Autodesk Inventor part; units mm, degrees
ref_plane "Arbeitsebene1" through (1.75, 0, 2.75) normal (0, 0, 1) x (1, 0, 0)
ref_plane "YZ Plane" through (0, 0, 0) normal (1, 0, 0) x (0, 1, 0)
ref_plane "XZ Plane" through (0, 0, 0) normal (0, 1, 0) x (-1, 0, 0)
sketch "Skizze1" plane through (0, 0, 0) normal (0, 0, 1) x (1, 0, 0)
  line L0 (-3.4, 0) -> (20.4, 0)
  line L1 (0, -0.55) -> (0, 3.3)
  line L2 (0, 2.75) -> (3.5, 2.75)
  line L3 (3.5, 2.75) -> (3.5, 2.5)
  line L4 (3.5, 2.5) -> (17, 2.5)
  line L5 (17, 2.5) -> (17, 0)
  line L6 (17, 0) -> (0, 0)
  line L7 (0, 0) -> (0, 2.75)
  dimension "d0" = 5.5
  dimension "d1" = 5
  dimension "d2" = 3.5
  dimension "d3" = 17
revolve "Umdrehung1" add sketch "Skizze1" angle 360 about axis through (-10, 0, 0) along (1, 0, 0)
hole "Bohrung1" at (0, 0, 0) direction (1, 0, 0) diameter 3 depth 6 tip angle 118
ref_plane "Arbeitsebene1" through (1.75, 0, 2.75) normal (0, 0, 1) x (1, 0, 0)
sketch "Skizze2" plane through (1.75, 0, 2.75) normal (0, 0, 1) x (1, 0, 0)
  line L0 (-5.15, 0) -> (18.65, 0)
  line L1 (-1.75, -3.85) -> (-1.75, 3.85)
  point P0 (-1.75, 0)
  point P1 (0, 0)
  dimension "d14" = 1.75
hole "Bohrung2" at (1.75, 0, 2.75) direction (0, 0, -1) diameter 1.567 end up to surface
properties part number "13_1087_027"
The listing builds one solid part. Answer for the finished solid, in the listing's coordinates (mm). A direction names the side the tool comes from. Round coordinates to 2 decimals unless told otherwise and drop trailing zeros. Write each loop counter-clockwise with the first axis right and the second up, starting at its lowest first coordinate (ties: lowest second). Pieces come first, ordered by that corner, then holes. Notation, with made-up numbers: (-6, 87) -> (32, 87) arc R12 ccw to (32, 109) -> close; hole circle Ø3 at (47.5, -1.75). An arc over 180 degrees is marked (long way). Write item = value, one per line.
1) Which of the six approach directions +Z, -Z, +X, -X, +Y, -Y give full straight-line access (tool end or side, diameter ignored) to faces 1 (the cylindrical face through (3.04, -0.07, -1.5)), 2 (the flat face through (17, 0, 0)), 3 (the cylindrical face through (2.445, -0.362, 2.004))?
Check values:
face_1 = -X
face_2 = +Z, -Z, +X, +Y, -Y
face_3 = +Z
2) Section A-A on z = 2.05 is taken. Write down the section's boundary in (x, y).
Check values:
outline = (0, -1.83) -> (3.5, -1.83) -> (3.5, -1.43) -> (17, -1.43) -> (17, 1.43) -> (3.5, 1.43) -> (3.5, 1.83) -> (0, 1.83) -> close; hole circle Ø1.57 at (1.75, 0)
3) Given pin 1 (1 mm diameter, centred on x = 7, z = 1.5, fed in from -Y); pin 2 (1.4 mm diameter, centred on x = 1.75, y = 0, fed in from +Z); pin 3 (1 mm diameter, centred on x = 3, z = -0.5, fed in from -Y), each flat-ended and moving along its own axis, determine where each tip first touches the part or whether it passes through.
Check values:
pin_1 = -2.29
pin_2 = -1.33
pin_3 = -2.75
4) Straight lines are drawn through the part: line 1 along X through (y, z) = (0, 1.85); line 2 along Z through (x, y) = (3, 0); line 3 along Z through (x, y) = (15.5, 0.1). For each, find the intervals that lie inside material, in ascending order. Write a range as [from, to].
Check values:
line_1 = [0, 0.97], [2.53, 17]
line_2 = [-2.75, -1.5], [1.5, 2.75]
line_3 = [-2.5, 2.5]
5) For a pull along Z with two mould halves and no side action, classify faces 4 (the cylindrical face through (10.34, -0.54, -2.44)), 5 (the flat face through (0, 1.2, -1.2)), 6 (the conical face through (6.745, -0.254, -0.056)) as released by +Z, released by -Z, zero draft, split by the parting line, or undercut.
Check values:
face_4 = split by the parting line
face_5 = zero draft
face_6 = undercut
6) Section C-C on x = 4.25 is taken. Write down the section's boundary in (y, z), plus the area to 3 significant figures.
Check values:
outline = circle Ø5 at (0, 0); hole circle Ø3 at (0, 0)
area = 12.6 mm²
7) Section B-B on y = 1.7 is taken. Write down the section's boundary in (x, z).
Check values:
outline = (0, -2.16) -> (3.5, -2.16) -> (3.5, -1.83) -> (17, -1.83) -> (17, 1.83) -> (3.5, 1.83) -> (3.5, 2.16) -> (0, 2.16) -> close
